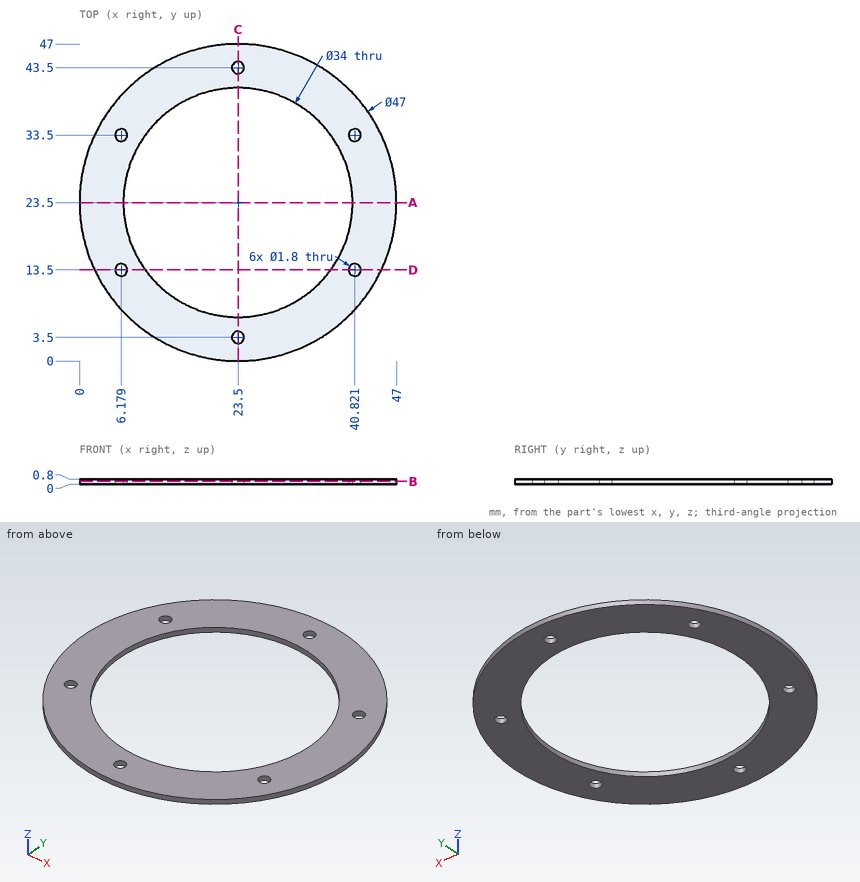
Job drawing, mm, ordinate dimensions from the low corner. One solid piece. Coordinates: 2 decimals unless noted, no trailing zeros. Order: outer loops, then holes, each group sorted by start corner. A loop starts at its lowest first (then second) coordinate and runs counter-clockwise, first axis right, second up. Notation, with made-up numbers: (-14, 78) -> (29, 78) arc R30 cw to (29, 103) -> close; hole circle Ø1 at (17.25, 77). An arc over 180 degrees is marked (long way). Put each result on its own line as item: value. Start each with the question number.
(1) Band-saw the part on D-D (y = 13.5). Give the cut face in (x, z).
(2) Band-saw the part on C-C (x = 23.5). Give the cut face in (y, z).
(3) Band-saw the part on A-A (y = 23.5). Give the cut face in (x, z), then the cut area to 3 significant figures.
(4) Probe line 1 along Y through (x, z) = (23.5, 0.45); line 2 along X through (y, z) = (37, 0.15) (1 decimal); line 3 along X through (y, z) = (8.5, 0.4). List the from-to ranges inside material, lowest first. Write a range as [from, to].
(5) Pin check, flat tip, straight feed: pin 1 Ø2.5 at (x, y) = (23.5, 43.5) entering from -Z. Stop position of the tip, or through.
(6) Band-saw the part on B-B (z = 0.45). Give the cut face in (x, y).
Determined:
1. outline: (2.23, 0) -> (5.28, 0) -> (5.28, 0.8) -> (2.23, 0.8) -> close; (7.08, 0) -> (9.75, 0) -> (9.75, 0.8) -> (7.08, 0.8) -> close; (37.25, 0) -> (39.92, 0) -> (39.92, 0.8) -> (37.25, 0.8) -> close; (41.72, 0) -> (44.77, 0) -> (44.77, 0.8) -> (41.72, 0.8) -> close
2. outline: (0, 0) -> (2.6, 0) -> (2.6, 0.8) -> (0, 0.8) -> close; (4.4, 0) -> (6.5, 0) -> (6.5, 0.8) -> (4.4, 0.8) -> close; (40.5, 0) -> (42.6, 0) -> (42.6, 0.8) -> (40.5, 0.8) -> close; (44.4, 0) -> (47, 0) -> (47, 0.8) -> (44.4, 0.8) -> close
3. outline: (0, 0) -> (6.5, 0) -> (6.5, 0.8) -> (0, 0.8) -> close; (40.5, 0) -> (47, 0) -> (47, 0.8) -> (40.5, 0.8) -> close
3. area: 10.4 mm²
4. line 1: y = [0, 2.6], [4.4, 6.5], [40.5, 42.6], [44.4, 47]
4. line 2: x = [4.3, 13.2], [33.8, 42.7]
4. line 3: x = [5.41, 15.5], [31.5, 41.59]
5. pin 1: stops at z = 0
6. outline: circle Ø47 at (23.5, 23.5); hole circle Ø1.8 at (6.18, 13.5); hole circle Ø1.8 at (6.18, 33.5); hole circle Ø34 at (23.5, 23.5); hole circle Ø1.8 at (23.5, 3.5); hole circle Ø1.8 at (23.5, 43.5); hole circle Ø1.8 at (40.82, 13.5); hole circle Ø1.8 at (40.82, 33.5)
